The drawing under review shows one solid part. Ordinate dimensions are in mm from its lowest x, y, z. A direction names the side the tool comes from. Give positions to 0.01 mm unless a question says otherwise; leave off trailing zeros. Order: outer loops, then holes, each group sorted by start corner. A loop starts at its lowest first (then second) coordinate and runs counter-clockwise, first axis right, second up. Notation, with made-up numbers: (41.25, 53.25) - (71.25, 53.25) arc R12 cw to (71.25, 71.25) - close; hole circle Ø1 at (-39, -12.75). An arc over 180 degrees is marked (long way). Use CSV: the item, a comma, the result in double quotes. Start each with the question number.
1. Take a section at B-B, the plane x = 6.25. State the section outline as (y, z) points.
2. Take a section at D-D, the plane z = 0.4. State the section outline as (x, y) points.
3. Take a section at A-A, the plane z = 1.7. State the section outline as (x, y) points.
4. For pin 1 (1 mm diameter, centred on x = 7, y = 1, fed in from +Z); pin 2 (0.8 mm diameter, centred on x = 11.5, y = 2.5, fed in from -Z); pin 3 (1 mm diameter, centred on x = 4.5, z = 3, fed in from +Y), all flat-tipped, find the tip position at first contact; note any pin that passes through.
5. Machinability: for the marked faces 1, 2 and 3, which of the approach directions +Z, -Z, +X, -X, +Y, -Y give a long, thin tool a straight path to every point of the face, cutting with its end or side? Answer none if there is none.
6. Take a section at C-C, the plane y = 2.5. State the section outline as (x, z) points.
7. To check wall thickness, follow line 1 (Y direction, x = 10.75, z = 0.4); line 2 (Z direction, x = 9.5, y = 1.9); line 3 (Z direction, x = 11.15, y = 2.5). State the ranges of each line that lie inside material, in increasing order. Write a range as [from, to].
8. Draft analysis for pull direction Y (two halves, no side actions). For the marked faces 4, 5 and 6, state which applies: released by +Y, released by -Y, zero draft, split by the parting line, or undercut.
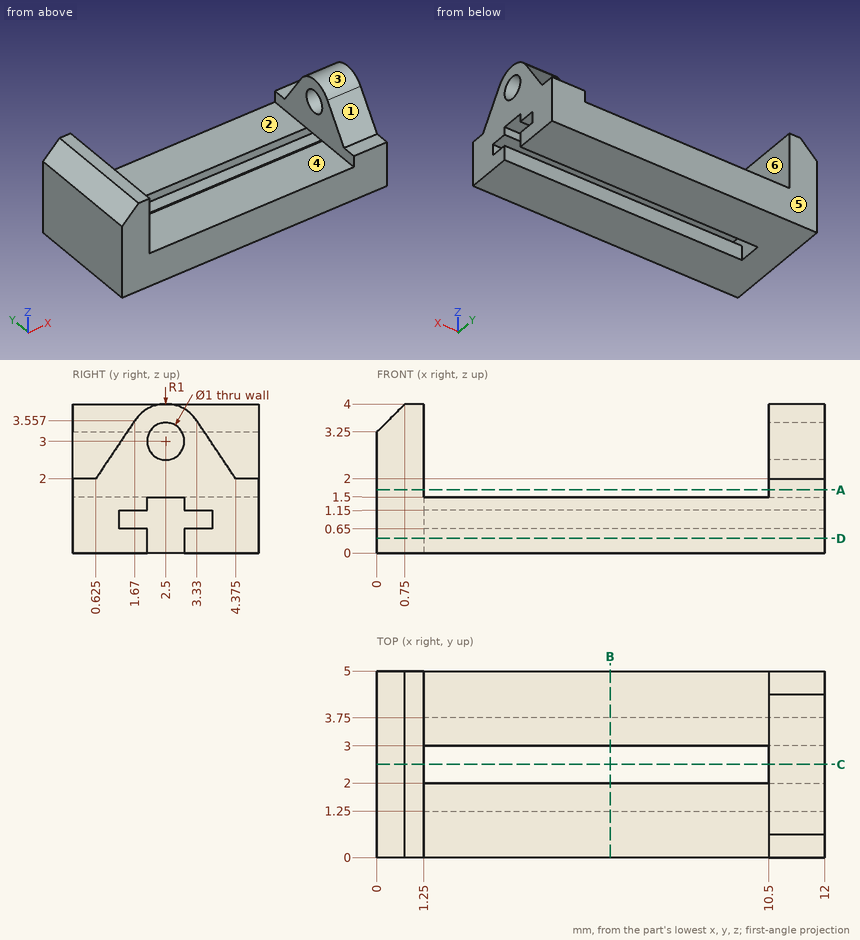
Determined:
1,outline,"(0, 0) - (2, 0) - (2, 0.65) - (1.25, 0.65) - (1.25, 1.15) - (2, 1.15) - (2, 1.5) - (0, 1.5) - close; (3, 0) - (5, 0) - (5, 1.5) - (3, 1.5) - (3, 1.15) - (3.75, 1.15) - (3.75, 0.65) - (3, 0.65) - close"
2,outline,"(0, 0) - (12, 0) - (12, 2) - (1.25, 2) - (1.25, 3) - (12, 3) - (12, 5) - (0, 5) - close"
3,outline,"(0, 0) - (1.25, 0) - (1.25, 5) - (0, 5) - close; (10.5, 0) - (12, 0) - (12, 5) - (10.5, 5) - close"
4,pin 1,"stops at z = 1.5"
4,pin 2,"stops at z = 1.5"
4,pin 3,"passes through"
5,face 1,"+Z, +X, -Y"
5,face 2,"+Z, +Y, -Y"
5,face 3,"+Z, +X"
6,outline,"(0, 0) - (1.25, 0) - (1.25, 4) - (0.75, 4) - (0, 3.25) - close; (10.5, 1.5) - (12, 1.5) - (12, 2.5) - (10.5, 2.5) - close; (10.5, 3.5) - (12, 3.5) - (12, 4) - (10.5, 4) - close"
7,line 1,"y = [0, 2], [3, 5]"
7,line 2,"z = [0, 0.65], [1.15, 1.5]"
7,line 3,"z = [1.5, 2.5], [3.5, 4]"
8,face 4,"zero draft"
8,face 5,"released by +Y"
8,face 6,"undercut"
